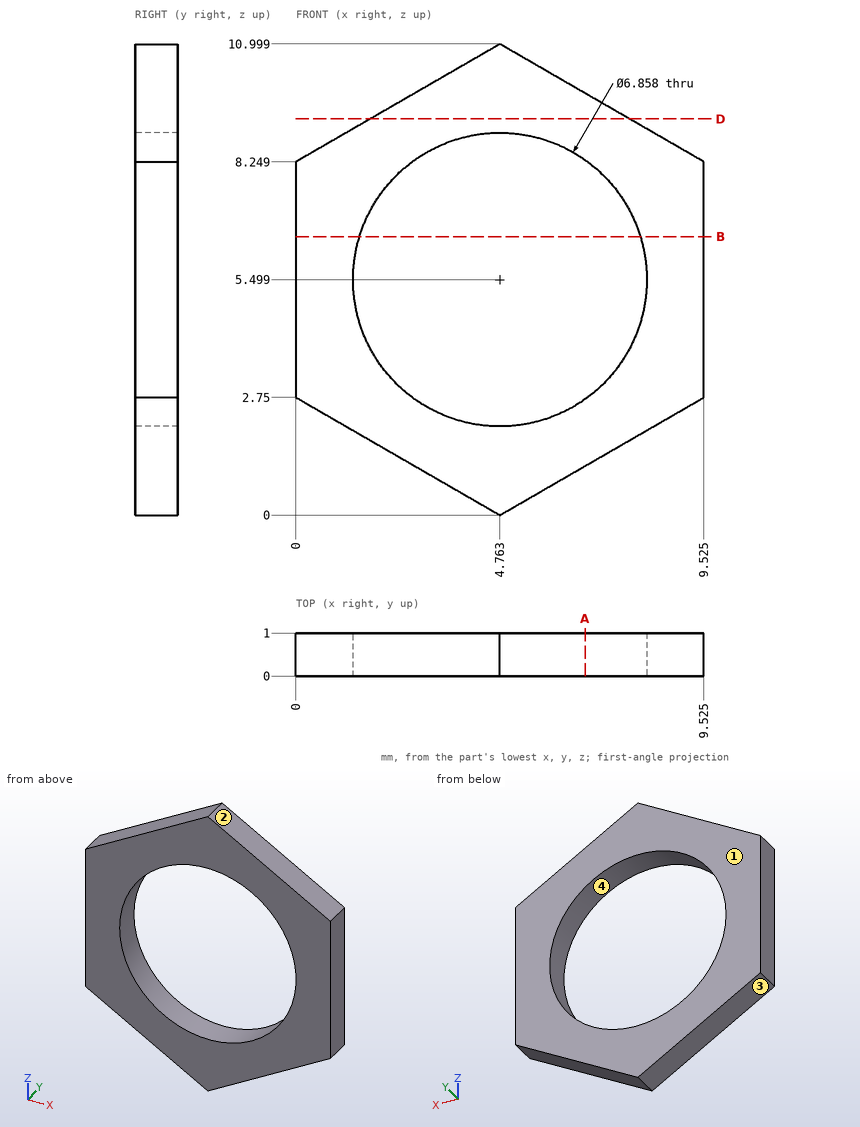
Part print with two shaded views. Sizes in mm from the minimum x, y, z corner. Round coordinates to 2 decimals unless told otherwise and drop trailing zeros. Loops run counter-clockwise (first coordinate to the right, second up) from the corner with the lowest first, then second, coordinate; pieces in that order, holes last.
Item 1: Drill centre lines: line 1 along X through (y, z) = (0.2, 7.5) (1 decimal); line 2 along X through (y, z) = (0.4, 6) (1 decimal); line 3 along Z through (x, y) = (6, 0.35) (1 decimal). Where is each one in solid material? Low to high.
Item 2: Saw through at B-B (z = 6.5). List the corners of the cut face in (x, y) (1 decimal).
Item 3: Saw through at A-A (x = 6.75). List the corners of the cut face in (y, z) (1 decimal).
Item 4: Two-plate mould, pull along X, no slides. Class the marked faces 1, 2, 3 and 4: released by +X, released by -X, zero draft, split by the parting line, or undercut.
Item 5: Saw through at D-D (z = 9.25). List the corners of the cut face in (x, y).
Worked answers:
1. line 1: x = 0 to 2, 7.5 to 9.5
1. line 2: x = 0 to 1.4, 8.2 to 9.5
1. line 3: z = 0.7 to 2.3, 8.7 to 10.3
2. outline: (0, 0) - (1.5, 0) - (1.5, 1) - (0, 1) - close; (8, 0) - (9.5, 0) - (9.5, 1) - (8, 1) - close
3. outline: (0, 1.1) - (1, 1.1) - (1, 2.7) - (0, 2.7) - close; (0, 8.3) - (1, 8.3) - (1, 9.9) - (0, 9.9) - close
4. face 1: zero draft
4. face 2: released by +X
4. face 3: released by -X
4. face 4: undercut
5. outline: (1.73, 0) - (7.79, 0) - (7.79, 1) - (1.73, 1) - close
